```python
from build123d import *

# Parameters (mm, degrees)
F0_R     = 12.25
F1_DEPTH = 42.5
F2_R     = 12.25
F2_R_2   = 10.5
F3_DEPTH = 2.5
F4_R     = 9.5
F5_DEPTH = 12.5
F6_R     = 10
F7_DEPTH = 18
F8_R     = 8.5
F9_DEPTH = 25


with BuildPart() as f1:
    # F0 (on Front) → F1 (new body)
    with BuildSketch(Plane.XZ):
        Circle(F0_R)
    extrude(amount=F1_DEPTH)

    # F2 (on face) → F3 (cut)
    with BuildSketch(Plane.XZ.offset(42.5)):
        Circle(F2_R)
        Circle(F2_R_2, mode=Mode.SUBTRACT)
    extrude(amount=-F3_DEPTH, mode=Mode.SUBTRACT)

    # F4 (on face) → F5 (cut)
    with BuildSketch(Plane.XZ.offset(42.5)):
        Circle(F4_R)
    extrude(amount=-F5_DEPTH, mode=Mode.SUBTRACT)

    # F6 (on face) → F7 (cut)
    with BuildSketch(Plane(origin=(0, 0, 0), x_dir=(-1, 0, 0), z_dir=(0, 1, 0))):
        Circle(F6_R)
    extrude(amount=-F7_DEPTH, mode=Mode.SUBTRACT)

    # F8 (on face) → F9 (cut)
    with BuildSketch(Plane(origin=(0, -18, 0), x_dir=(-1, 0, 0), z_dir=(0, 1, 0))):
        Circle(F8_R)
    extrude(amount=-F9_DEPTH, mode=Mode.SUBTRACT)


solid = f1.part
```
Geometry check sheet. Reference: the model listing, model coordinates, mm. A direction names the side the tool comes from. Coordinates: 2 decimals unless noted, no trailing zeros. Order: outer loops, then holes, each group sorted by start corner. A loop starts at its lowest first (then second) coordinate and runs counter-clockwise, first axis right, second up. Notation, with made-up numbers: M 50,26 L 105,26 A20 cw 105,58 Z; hole C 59,87 d7. An arc over 180 degrees is marked long. One line per question, with ' | ' between items. Start each with the question number.
Item 1: Cross-section at A-A on x = 0. Enter the section's corners in (y, z), then the cut area to 3 significant figures.
Item 2: Draft check along X on faces 1 (the cylindrical face through (10, -41.3, 3.2)), 2 (the cylindrical face through (4.38, -36.34, -8.43)), 3 (the flat face through (9, -40, 6)). Enter one of: pulls with the +X half, pulls with the -X half, needs draft (parallel to the pull), parting line crosses it, or undercut.
Item 3: Gauge pin test, flat ends, axial feed: pin 1 (1 mm diameter, centred on y = -10.5, z = -4.5, fed in from -X); pin 2 (4 mm diameter, centred on x = -5, y = -31, fed in from +Z); pin 3 (7.5 mm diameter, centred on x = 1, z = -4.5, fed in from -Y); pin 4 (8 mm diameter, centred on x = 8, y = -7.5, fed in from -Z). Record the tip position at first contact, or that the pin passes through.
Item 4: Material ranges on L1, parallel to Z at x = 0, y = -8; L2, parallel to Z at x = 0, y = -24.5; L3, parallel to X at y = -13, z = 5.5, recorded low to high. Write a range as [from, to].
Item 5: Set-up check for faces 4 (the cylindrical face through (2.17, -8.87, -9.76)), 5 (the flat face through (-2.2, -30, -8.4)), 6 (the cylindrical face through (6.586, -19.72, 10.329)): record each of +Z, -Z, +X, -X, +Y, -Y from which the full face is reachable in a straight line by a thin tool's end or side.
Item 6: Cross-section at C-C on y = -20. Enter the section's corners in (x, z).
Item 7: Cross-section at B-B on z = 0. Enter the section's corners in (x, y).
Findings:
1) outline: M -42.5,-10.5 L -40,-10.5 L -40,-12.25 L 0,-12.25 L 0,-10 L -18,-10 L -18,-8.5 L -30,-8.5 L -30,-9.5 L -42.5,-9.5 Z; M -42.5,9.5 L -30,9.5 L -30,8.5 L -18,8.5 L -18,10 L 0,10 L 0,12.25 L -40,12.25 L -40,10.5 L -42.5,10.5 Z | area: 231 mm²
2) face 1: parting line crosses it | face 2: undercut | face 3: needs draft
3) pin 1: stops at x = -11.58 | pin 2: stops at z = 11.88 | pin 3: passes through | pin 4: stops at z = -11.58
4) L1: z = [-12.25, -10], [10, 12.25] | L2: z = [-12.25, -8.5], [8.5, 12.25] | L3: x = [-10.95, -8.35], [8.35, 10.95]
5) face 4: +Y | face 5: -Y | face 6: +Y, -Y
6) outline: C 0,0 d24.5; hole C 0,0 d17
7) outline: M -12.25,-40 L -10.5,-40 L -10.5,-42.5 L -9.5,-42.5 L -9.5,-30 L -8.5,-30 L -8.5,-18 L -10,-18 L -10,0 L -12.25,0 Z; M 8.5,-30 L 9.5,-30 L 9.5,-42.5 L 10.5,-42.5 L 10.5,-40 L 12.25,-40 L 12.25,0 L 10,0 L 10,-18 L 8.5,-18 Z
